Geometry check sheet. Reference: the model listing, model coordinates, mm. Face numbers are marked on the shaded views. Coordinates: 2 decimals unless noted, no trailing zeros. Order: outer loops, then holes, each group sorted by start corner. A loop starts at its lowest first (then second) coordinate and runs counter-clockwise, first axis right, second up. Notation, with made-up numbers: (30, 32.25) - (74, 32.25) arc R26 cw to (74, 71.25) - close; hole circle Ø8 at (73, 84.5). An arc over 180 degrees is marked (long way). Return JSON: item names as keys, results as strings. Group by question number.
Item 1: Draft check along X on the marked faces 1 and 2. Enter one of: pulls with the +X half, pulls with the -X half, needs draft (parallel to the pull), parting line crosses it, or undercut.
Item 2: Scan lines: probe 1 along X at (y, z) = (-20.5, 2.2); probe 2 along X at (y, z) = (-24.75, 0.85); probe 3 along Z at (x, y) = (24, -22). Record each from-to range of solid material in increasing order.
Item 3: Gauge pin test, flat ends, axial feed: pin 1 (6.5 mm diameter, centred on x = 47.5, y = -20.5, fed in from +Z); pin 2 (2 mm diameter, centred on x = 41.5, z = 2, fed in from +Y); pin 3 (1.8 mm diameter, centred on x = -37.5, y = -19, fed in from +Z). Record the tip position at first contact, or that the pin passes through.
Item 4: Section check A-A on y = -19.5. Give the number of separate pieces and of enclosed holes in the cut face, then the cut area to 3 significant figures.
Item 5: Section check C-C on x = -31. Enter the section's corners in (y, z), then the cut area to 3 significant figures.
from build123d import *

# Parameters (mm, degrees)
F0_W      = 98
F0_H      = 13
F1_DEPTH  = 3
F2_R      = 3
F3_R      = 2
F4_DEPTH  = 20
F5_R      = 7.5
F6_DEPTH  = 4.75
F8_DEPTH  = 1.75
F9_W      = 25
F9_H      = 16
F10_DEPTH = 2
F11_F1_R  = 1
F11_F2_R  = 0.9999


# Not quite as in the source:
# - a fillet or chamfer is up to 0.001 mm smaller than in the source, because OpenCascade refuses the exact size


with BuildPart() as f1:
    # F0 (on Top) → F1 (new body)
    with BuildSketch(Plane.XY):
        with Locations((5.7567551136, -20.2820947109)):
            Rectangle(F0_W, F0_H)
    extrude(amount=F1_DEPTH)

    # F2
    f2_edges = [f1.edges().sort_by_distance(p)[0] for p in [
        (-43.243245, -13.782095, 1.5),
        (54.756755, -13.782095, 1.5),
    ]]
    fillet(f2_edges, radius=F2_R)

    # F3 (on face) → F4 (cut)
    with BuildSketch(Plane.XY.offset(3)):
        with Locations((48.7567551136, -20.5320947109)):
            Circle(F3_R)
        with Locations((-37.2432448864, -20.5320947109)):
            Circle(F3_R)
    extrude(amount=-F4_DEPTH, mode=Mode.SUBTRACT)

    # F5 (on Top) → F6 (join)
    with BuildSketch(Plane.XY):
        with Locations((5.7567551136, -18.2820947109)):
            Circle(F5_R)
    extrude(amount=F6_DEPTH)

    # F7 (on face) → F8 (cut)
    with BuildSketch(Plane.XY.offset(3)):
        Polygon((-33.7791432713, -20.5320947109), (-35.5111940788, -17.5320947109), (-38.975295694, -17.5320947109), (-40.7073465015, -20.5320947109), (-38.975295694, -23.5320947109), (-35.5111940788, -23.5320947109), align=None)
        Polygon((50.4888059212, -17.5320947109), (47.024704306, -17.5320947109), (45.2926534985, -20.5320947109), (47.024704306, -23.5320947109), (50.4888059212, -23.5320947109), (52.2208567287, -20.5320947109), align=None)
    extrude(amount=-F8_DEPTH, mode=Mode.SUBTRACT)

    # F9 (on face) → F10 (cut)
    with BuildSketch(Plane(origin=(0, 0, 0), x_dir=(1, 0, 0), z_dir=(0, 0, -1))):
        with Locations((5.7567551136, 18.7820947109)):
            Rectangle(F9_W, F9_H)
    extrude(amount=-F10_DEPTH, mode=Mode.SUBTRACT)

    # F11: fillet of radius 1 on 6 edges, made by hand

    # F11_f1
    f11_f1_edges = [f1.edges().sort_by_distance(p)[0] for p in [
        (18.2567551136, -20.2820947109, 2),
        (-6.7432448864, -20.2820947109, 2),
    ]]
    fillet(f11_f1_edges, radius=F11_F1_R)

    # F11_f2 (radius 1 in the source; OpenCascade refuses exactly that, so slightly less here)
    f11_f2_edges = [f1.edges().sort_by_distance(p)[0] for p in [
        (14.5067551136, -13.7820947109, 2),
        (5.7567551136, -10.7820947109, 2),
        (-2.9932448864, -13.7820947109, 2),
        (5.7567551136, -26.7820947109, 2),
        (17.9638618948, -26.7820947109, 1.7071067812),
        (-6.4503516676, -26.7820947109, 1.7071067812),
        (-6.4503516676, -13.7820947109, 1.7071067812),
        (17.9638618948, -13.7820947109, 1.7071067812),
    ]]
    fillet(f11_f2_edges, radius=F11_F2_R)


solid = f1.part
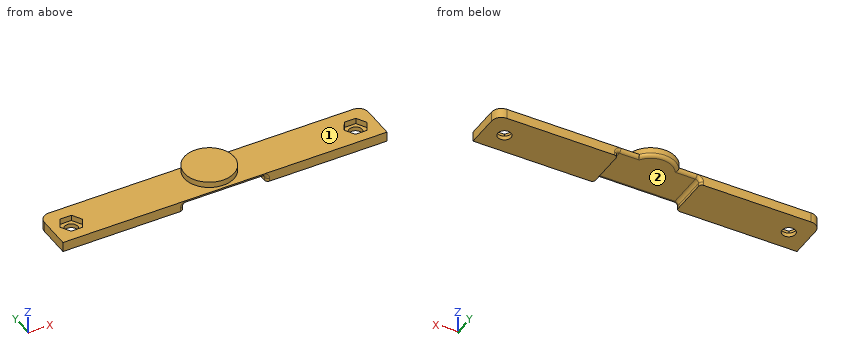
Computed:
{
 "1": {"face 1": "needs draft", "face 2": "undercut"},
 "2": {"probe 1": "x = -43.24 to -40.69, -33.8 to 45.31, 52.2 to 54.76", "probe 2": "x = -43.24 to -6.74, 18.26 to 54.76", "probe 3": "z = 0 to 3"},
 "3": {"pin 1": "stops at z = 3", "pin 2": "stops at y = -13.78", "pin 3": "stops at z = 1.25"},
 "4": {"separate pieces": "3", "enclosed holes": "0", "area": "242 mm²"},
 "5": {"outline": "(-26.78, 0) - (-13.78, 0) - (-13.78, 3) - (-26.78, 3) - close", "area": "39.0 mm²"}
}
